from build123d import *

# Parameters (mm, degrees)
SKETCH_W        = 64.8
SKETCH_H        = 50
PAD_DEPTH       = 50
POCKET_DEPTH    = 64.801
POCKET001_DEPTH = 64.801
POCKET002_DEPTH = 64.801
SKETCH004_W     = 60.8
SKETCH004_H     = 10.4
POCKET003_DEPTH = 30
POCKET004_DEPTH = 18.9853350022
POCKET005_DEPTH = 64.801


with BuildPart() as part:
    # Sketch → Pad (new body)
    with BuildSketch(Plane.XY):
        with Locations((32.4, 25)):
            Rectangle(SKETCH_W, SKETCH_H)
    extrude(amount=PAD_DEPTH)

    # Sketch001 → Pocket (cut, through all)
    with BuildSketch(Plane.YZ.offset(64.8)):
        Polygon((0, 0), (0, 50), (18.1985117133, 50), align=None)
    extrude(amount=-POCKET_DEPTH, mode=Mode.SUBTRACT)

    # Sketch002 → Pocket001 (cut, through all)
    with BuildSketch(Plane.YZ.offset(64.8)):
        Polygon((33.3985117133, 50), (18.8397023427, 10), (50, 10), (50, 50), align=None)
    extrude(amount=-POCKET001_DEPTH, mode=Mode.SUBTRACT)

    # Sketch003 → Pocket002 (cut, through all)
    with BuildSketch(Plane.YZ.offset(64.8)):
        Polygon((18.1985117133, 50), (31.620449481, 45.1148141664), (33.3985117133, 50), align=None)
    extrude(amount=-POCKET002_DEPTH, mode=Mode.SUBTRACT)

    # Sketch004 → Pocket003 (cut)
    with BuildSketch(Plane(origin=(0, 18.1985117133, 50), x_dir=(1, 0, 0), z_dir=(0, 0.3420201433, 0.9396926208))):
        with Locations((32.4, 7.0833278359)):
            Rectangle(SKETCH004_W, SKETCH004_H)
    extrude(amount=-POCKET003_DEPTH, mode=Mode.SUBTRACT)

    # Sketch005 → Pocket004 (cut, through all)
    with BuildSketch(Plane(origin=(0, 1.76974927, -0.6441360564), x_dir=(-1, 0, 0), z_dir=(0, 0.9396926208, -0.3420201433))):
        Polygon((-62.8, 32.2088886238), (-40.4, 32.2088886238), (-40.4, 23.2088886238), (-24.4, 23.2088886238), (-24.4, 32.2088886238), (-2, 32.2088886238), (-1.996389, 63.8506663486), (-62.8, 53.2088886238), align=None)
    extrude(amount=-POCKET004_DEPTH, mode=Mode.SUBTRACT)

    # Sketch006 → Pocket005 (cut, through all)
    with BuildSketch(Plane.YZ.offset(64.8)):
        Polygon((31.620449481, 45.1148141664), (16.420449481, 45.1148141664), (18.1985117133, 50), align=None)
    extrude(amount=-POCKET005_DEPTH, mode=Mode.SUBTRACT)


solid = part.part
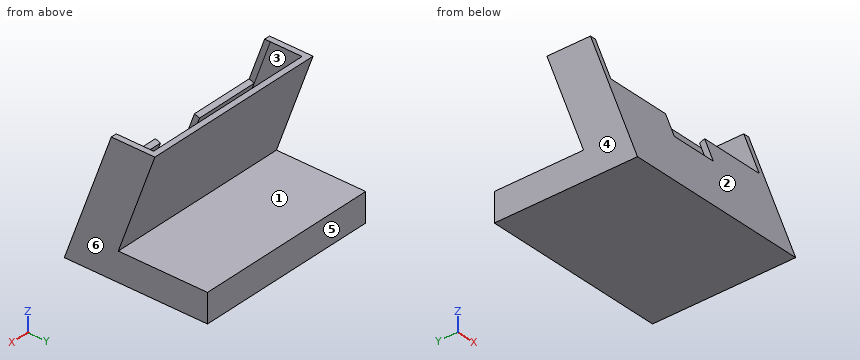
Can you work these out from the model? Positions are in its coordinate system, mm. Face numbers are marked on the shaded views. A direction names the side the tool comes from. Coordinates: 2 decimals unless noted, no trailing zeros. Write each loop counter-clockwise with the first axis right and the second up, starting at its lowest first coordinate (ties: lowest second). Pieces come first, ordered by that corner, then holes. Notation, with made-up numbers: (-14, 69) - (6, 69) arc R12 cw to (6, 80) - close; hole circle Ø4 at (10, -30). An arc over 180 degrees is marked (long way). Return JSON: item names as keys, results as strings. Group by question number.
Item 1: If we section it at A-A (x = 55.5): Write out the boundary of the cut face in (y, z).
Item 2: If we section it at D-D (y = 47.5): Write out the boundary of the cut face in (x, z), then the cut area to 3 significant figures.
Item 3: We'd pull the mould along X, two halves only. Please class the marked faces 3, 4, 5 and 6: pulls with the +X half, pulls with the -X half, needs draft (parallel to the pull), parting line crosses it, or undercut.
Item 4: If we section it at B-B (y = 21): Write out the boundary of the cut face in (x, z).
Item 5: Which directions (+Z, -Z, +X, -X, +Y, -Y) give clear straight access to the entire face, cutting with the end or side of a thin tool? Please do the marked faces 1 and 2.
Item 6: Please list where these lines run through material, in increasing order: probe 1 along X at (y, z) = (27, 39.5); probe 2 along Y at (x, z) = (46, 29.5); probe 3 along Z at (x, y) = (26.5, 35.5).
Item 7: I'm going to push flat-ended pins straight in: pin 1 Ø8 at (x, z) = (39.5, 32) entering from +Y; pin 2 Ø5.5 at (y, z) = (9, 26.5) entering from -X; pin 3 Ø2 at (x, z) = (23.5, 31.5) entering from +Y; pin 4 Ø8 at (x, z) = (42, 18.5) entering from +Y. Where does each tip first touch, or does it pass through?
Return value:
{
 "1": {"outline": "(0, 0) - (50, 0) - (50, 10) - (18.84, 10) - (31.62, 45.11) - (29.49, 45.11) - (19.48, 17.61) - (9.71, 21.17) - (12.79, 29.62) - (11.02, 30.27) - close"},
 "2": {"outline": "(0, 0) - (64.8, 0) - (64.8, 10) - (0, 10) - close", "area": "648 mm^2"},
 "3": {"face 3": "undercut", "face 4": "pulls with the -X half", "face 5": "needs draft", "face 6": "pulls with the +X half"},
 "4": {"outline": "(0, 0) - (64.8, 0) - (64.8, 10) - (0, 10) - close; (0, 15.94) - (64.8, 15.94) - (64.8, 45.11) - (62.8, 45.11) - (62.8, 21.78) - (2, 21.78) - (2, 45.11) - (0, 45.11) - close"},
 "5": {"face 1": "+X, -X, +Y", "face 2": "+Z, +X, -X, -Y"},
 "6": {"probe 1": "x = 0 to 2, 62.8 to 64.8", "probe 2": "y = 10.74 to 12.74, 23.81 to 25.94", "probe 3": "z = 0 to 10"},
 "7": {"pin 1": "stops at y = 28.3", "pin 2": "stops at x = 0", "pin 3": "stops at y = 27.03", "pin 4": "stops at y = 23.39"}
}
